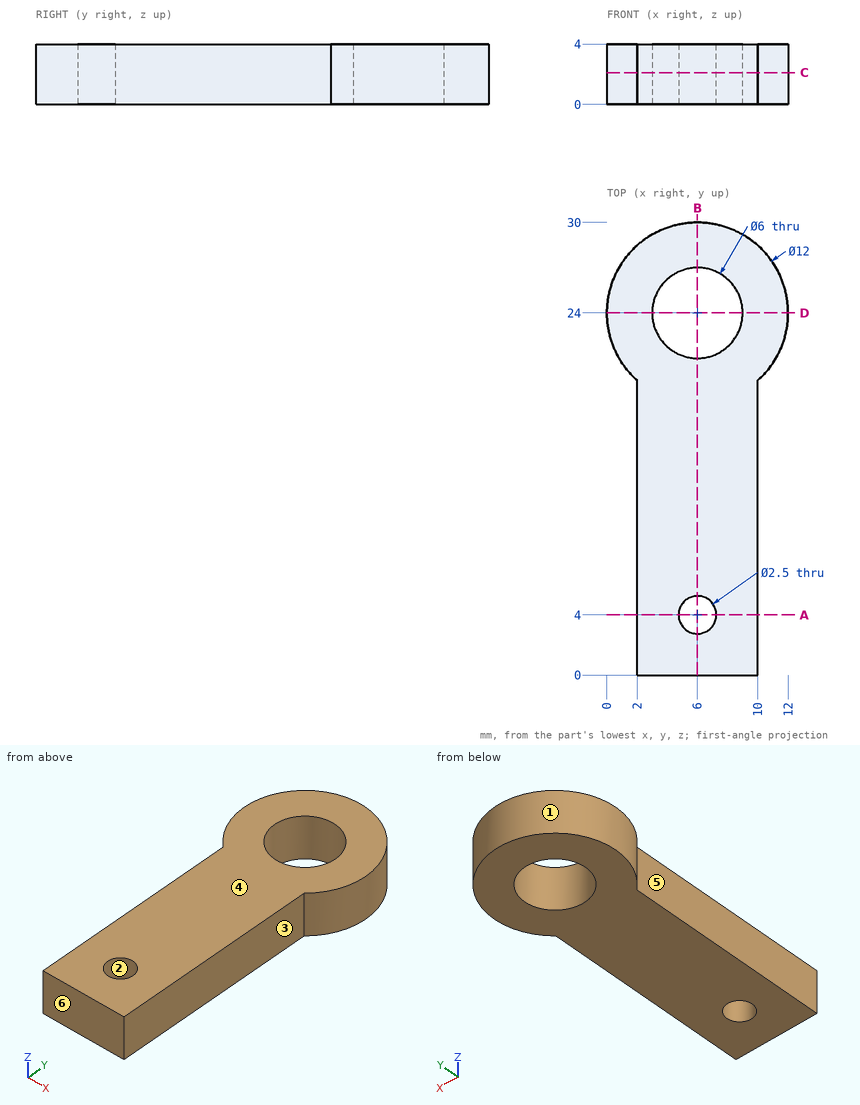
Could you check a few things on this drawing? It's one solid part, dimensions in mm from its lowest x, y, z. A direction names the side the tool comes from. Give positions to 0.01 mm unless a question says otherwise; leave off trailing zeros. Write each loop counter-clockwise with the first axis right and the second up, starting at its lowest first coordinate (ties: lowest second). Pieces come first, ordered by that corner, then holes. Notation, with made-up numbers: (73, 32) -> (99, 32) arc R30 ccw to (99, 65) -> close; hole circle Ø3 at (85.25, 81). An arc over 180 degrees is marked (long way). Answer as CSV lines item,"result". Start each with the question number.
(1) If we section it at C-C, the plane z = 2.1: Write out the boundary of the cut face in (x, y).
(2) Which directions (+Z, -Z, +X, -X, +Y, -Y) give clear straight access to the entire face, cutting with the end or side of a thin tool? Please do the marked faces 5 and 6.
(3) Please list where these lines run through material, in increasing order: line 1 (Y direction, x = 6, z = 2.2); line 2 (Y direction, x = 5, z = 1.1); line 3 (X direction, y = 4, z = 2.35).
(4) If we mould it in two halves opening along X, with no side actions, what happens to the marked faces 1, 2, 3 and 4? For each: +X half, -X half, draft (parallel to the pull), parting line (faces both ways), or undercut.
(5) If we section it at B-B, the plane x = 6: Write out the boundary of the cut face in (y, z), and give its area (3 significant figures).
(6) I'm going to push flat-ended pins straight in: pin 1 Ø1.5 at (x, z) = (5, 1) entering from -Y; pin 2 Ø1 at (y, z) = (3.5, 1.5) entering from +X; pin 3 Ø2 at (y, z) = (14, 2) entering from -X. Where does each tip first touch, or does it pass through?
(7) If we section it at A-A, the plane y = 4: Write out the boundary of the cut face in (x, z).
(8) If we section it at D-D, the plane y = 24: Write out the boundary of the cut face in (x, z), and give its area (3 significant figures).
Answer list:
1,outline,"(2, 0) -> (10, 0) -> (10, 19.53) arc R6 ccw (long way) to (2, 19.53) -> close; hole circle Ø6 at (6, 24); hole circle Ø2.5 at (6, 4)"
2,face 5,"+Z, -Z, -X, -Y"
2,face 6,"+Z, -Z, +X, -X, -Y"
3,line 1,"0 to 2.75, 5.25 to 21, 27 to 30"
3,line 2,"0 to 3.25, 4.75 to 21.17, 26.83 to 29.92"
3,line 3,"2 to 4.75, 7.25 to 10"
4,face 1,"parting line"
4,face 2,"undercut"
4,face 3,"+X half"
4,face 4,"draft"
5,outline,"(0, 0) -> (2.75, 0) -> (2.75, 4) -> (0, 4) -> close; (5.25, 0) -> (21, 0) -> (21, 4) -> (5.25, 4) -> close; (27, 0) -> (30, 0) -> (30, 4) -> (27, 4) -> close"
5,area,"86.0 mm^2"
6,pin 1,"y = 0"
6,pin 2,"x = 10"
6,pin 3,"x = 2"
7,outline,"(2, 0) -> (4.75, 0) -> (4.75, 4) -> (2, 4) -> close; (7.25, 0) -> (10, 0) -> (10, 4) -> (7.25, 4) -> close"
8,outline,"(0, 0) -> (3, 0) -> (3, 4) -> (0, 4) -> close; (9, 0) -> (12, 0) -> (12, 4) -> (9, 4) -> close"
8,area,"24.0 mm^2"
